Design review of the part shown in the three views and the two pictorial views. Dimensions are in mm from the part's minimum x, y and z. Give positions to 0.01 mm unless a question says otherwise; leave off trailing zeros. Order: outer loops, then holes, each group sorted by start corner. A loop starts at its lowest first (then second) coordinate and runs counter-clockwise, first axis right, second up. Notation, with made-up numbers: (62.5, 87) - (71.5, 87) arc R20 ccw to (71.5, 122) - close; hole circle Ø4 at (21, 77.5). An arc over 180 degrees is marked (long way). Put each result on its own line as item: value. Start each with the question number.
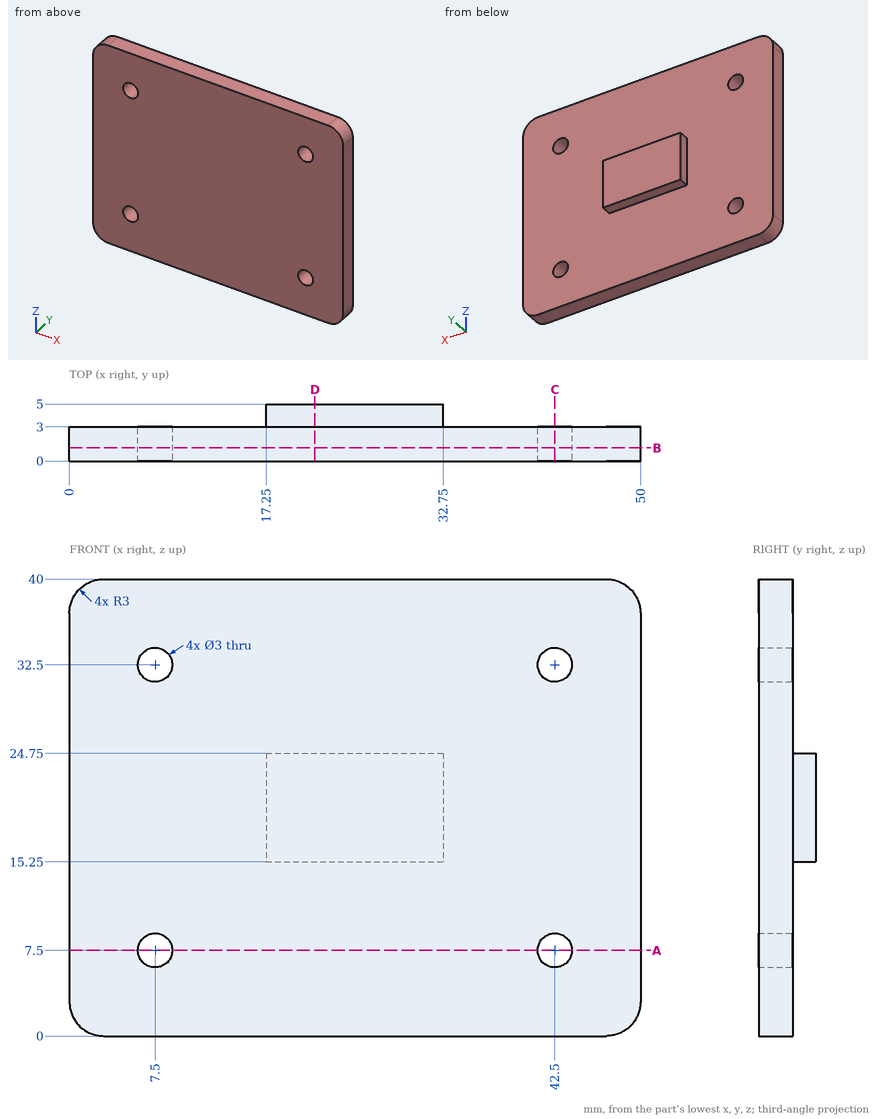
1. Add section C-C, the plane x = 42.5. Give the boundary of the cut face in (y, z).
2. Add section A-A, the plane z = 7.5. Give the boundary of the cut face in (x, y).
3. Add section D-D, the plane x = 21.5. Give the boundary of the cut face in (y, z).
4. Add section B-B, the plane y = 1.15. Give the boundary of the cut face in (x, z), then the cut area to 3 significant figures.
5. Clearance check with flat-ended pins moving along their axes: pin 1 (2 mm diameter, centred on x = 11, z = 11, fed in from +Y); pin 2 (1 mm diameter, centred on x = 26.5, y = 4.5, fed in from +Z); pin 3 (2.5 mm diameter, centred on x = 42.5, z = 32.5, fed in from +Y); pin 4 (2 mm diameter, centred on y = 4.5, z = 22.5, fed in from -X). State where each tip first meets the part, or that it passes through.
6. Wall thickness on line 1 (X direction, y = 1.65, z = 7.5); line 2 (Z direction, x = 42.5, y = 2.25); line 3 (Y direction, x = 11.5, z = 33): over which ranges is each line inside the solid? List them lowest first. Write a range as from..to.
Found:
1. outline: (0, 0) - (3, 0) - (3, 6) - (0, 6) - close; (0, 9) - (3, 9) - (3, 31) - (0, 31) - close; (0, 34) - (3, 34) - (3, 40) - (0, 40) - close
2. outline: (0, 0) - (6, 0) - (6, 3) - (0, 3) - close; (9, 0) - (41, 0) - (41, 3) - (9, 3) - close; (44, 0) - (50, 0) - (50, 3) - (44, 3) - close
3. outline: (0, 0) - (3, 0) - (3, 15.25) - (5, 15.25) - (5, 24.75) - (3, 24.75) - (3, 40) - (0, 40) - close
4. outline: (0, 3) arc R3 ccw to (3, 0) - (47, 0) arc R3 ccw to (50, 3) - (50, 37) arc R3 ccw to (47, 40) - (3, 40) arc R3 ccw to (0, 37) - close; hole circle Ø3 at (7.5, 7.5); hole circle Ø3 at (7.5, 32.5); hole circle Ø3 at (42.5, 7.5); hole circle Ø3 at (42.5, 32.5)
4. area: 1,960 mm^2
5. pin 1: stops at y = 3
5. pin 2: stops at z = 24.75
5. pin 3: passes through
5. pin 4: stops at x = 17.25
6. line 1: x = 0..6, 9..41, 44..50
6. line 2: z = 0..6, 9..31, 34..40
6. line 3: y = 0..3
